Design review of the part built by this model. Coordinates are the model's own, in mm. Face numbers are marked on the shaded views. Coordinates: 2 decimals unless noted, no trailing zeros. Loops run counter-clockwise (first coordinate to the right, second up) from the corner with the lowest first, then second, coordinate; pieces in that order, holes last. Notation, with made-up numbers: (-37.75, 38) - (-2.75, 38) arc R18 ccw to (-2.75, 44) - close; hole circle Ø8 at (86, -18). An arc over 180 degrees is marked (long way). Return JSON: item names as keys, results as strings. Group by question number.
from build123d import *

# Parameters (mm, degrees)
SKETCH_1_R      = 7
SKETCH_1_R_2    = 4
EXTRUDE_1_DEPTH = 4
SKETCH_2_W      = 2
SKETCH_2_H      = 1.5
FILLET_1_R      = 0.5


with BuildPart() as part:
    # 草图1 → 凸台-拉伸1 (new body)
    with BuildSketch(Plane.XY):
        Circle(SKETCH_1_R)
        Circle(SKETCH_1_R_2, mode=Mode.SUBTRACT)
    extrude(amount=EXTRUDE_1_DEPTH)

    # 草图2 → 切除-旋转1 (revolve, cut)
    with BuildSketch(Plane(origin=(0, 0, 0), x_dir=(0, 0, -1), z_dir=(1, 0, 0)), mode=Mode.PRIVATE) as cut_revolve_1_sk:
        with Locations((-2, 6.25)):
            Rectangle(SKETCH_2_W, SKETCH_2_H)
    revolve(cut_revolve_1_sk.sketch.rotate(Axis((0, 0, -1.510874211), (0, 0, 1)), 90), axis=Axis((0, 0, -1.510874211), (0, 0, 1)), mode=Mode.SUBTRACT)

    # 圆角1
    fillet_1_edges = [part.edges().sort_by_distance(p)[0] for p in [
        (-7, 0, 1),
        (-7, 0, 3),
        (-7, 0, 0),
        (-7, 0, 4),
    ]]
    fillet(fillet_1_edges, radius=FILLET_1_R - 0.0001)  # a hair under: the kernel refuses the full size


solid = part.part
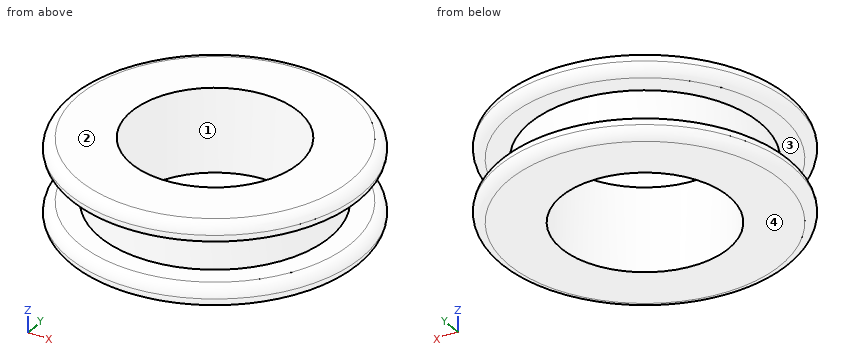
Item 1: Draft analysis for pull direction Z (two halves, no side actions). For the marked faces 1, 2, 3 and 4, state which applies: pulls with the +Z half, pulls with the -Z half, needs draft (parallel to the pull), parting line crosses it, or undercut.
Item 2: Add section C-C (z = 1.65). State the section outline as (x, y) points.
Item 3: To check wall thickness, follow line 1 (Z direction, x = -1.25, y = 5.75); line 2 (Y direction, x = 0, z = 2.25); line 3 (X direction, y = -2.5, z = 0.85). State the ranges of each line that lie inside material, in increasing order. Write a range as from..to.
Item 4: For P1, Ø2, axis at y = 2.5, z = 0.5, coming from the -X side; P2, Ø8, axis at x = 3.5, y = 1, coming from the +Z side; P3, Ø5, axis at x = 0, y = 0, coming from the -Z side, all flat-tipped, find the tip position at first contact; note any pin that passes through.
Answers below:
{
 "1": {"face 1": "needs draft", "face 2": "pulls with the +Z half", "face 3": "undercut", "face 4": "pulls with the -Z half"},
 "2": {"outline": "circle Ø11 at (0, 0); hole circle Ø8 at (0, 0)"},
 "3": {"line 1": "z = 0..1, 3..4", "line 2": "y = -5.5..-4, 4..5.5", "line 3": "x = -6.39..-3.12, 3.12..6.39"},
 "4": {"P1": "stops at x = -6.84", "P2": "stops at z = 4", "P3": "passes through"}
}
